Autodesk Inventor part; units mm, degrees
ref_plane "YZ Plane" through (0, 0, 0) normal (1, 0, 0) x (0, 1, 0)
ref_plane "XZ Plane" through (0, 0, 0) normal (0, 1, 0) x (-1, 0, 0)
ref_plane "XY Plane" through (0, 0, 0) normal (0, 0, 1) x (1, 0, 0)
sketch "Sketch1" plane through (0, 0, 0) normal (0, 0, 1) x (1, 0, 0)
  circle A0 centre (0, 0) radius 10
  circle A1 centre (0, 0) radius 20
  line L0 (-15, 0) -> (15, 0)
  line L1 (15, 0) -> (15, 50)
  line L2 (15, 50) -> (-15, 50)
  line L3 (-15, 50) -> (-15, 0)
  point P0 (-15, 13.2288)
  point P1 (15, 13.2288)
  dimension "d0" = 20
  dimension "d1" = 40
  dimension "d2" = 30
  dimension "d3" = 50
extrude "Extrusion1" add sketch "Sketch1" along normal blind 20
sketch "Sketch2" plane through (0, 0, 20) normal (0, 0, 1) x (1, 0, 0)
  circle A0 centre (0, 0) radius 10
  dimension "d6" = 20
extrude "Extrusion2" cut sketch "Sketch2" against normal blind 15
sketch "Sketch4" plane through (-15, 13.2288, 0) normal (-1, 0, 0) x (0, 0, 1)
  line L0 (0, 36.7712) -> (20, 36.7712)
  line L1 (0, 0) -> (0, 36.7712)
  line L2 (20, 36.7712) -> (0, 36.7712)
  line L3 (0, 36.7712) -> (0, 0)
  line L4 (0, 0) -> (20, 0)
  line L5 (20, 0) -> (20, 36.7712)
  line L6 (0, 0) -> (20, 0)
  line L7 (20, 36.7712) -> (10, 36.7712)
  line L8 (10, 36.7712) -> (10, 0)
  line L9 (10, 0) -> (20, 0)
  line L10 (20, 0) -> (20, 36.7712)
  line L11 (10, 0) -> (16, 0)
  line L12 (16, 0) -> (16, 25)
  line L13 (16, 25) -> (10, 25)
  line L14 (10, 25) -> (10, 0)
  line L15 (10, 25) -> (4, 25)
  line L16 (4, 25) -> (4, 0)
  line L17 (4, 0) -> (10, 0)
  line L18 (10, 0) -> (10, 25)
  line L19 (4, 25) -> (16, 25)
  line L20 (16, 25) -> (16, 30.0005)
  line L21 (16, 30.0005) -> (4, 30.0005)
  line L22 (4, 30.0005) -> (4, 25)
  line L23 (4, 30.0005) -> (16, 30.0005)
  line L24 (16, 30.0005) -> (16, 7.0005)
  line L25 (16, 7.0005) -> (4, 7.0005)
  line L26 (4, 7.0005) -> (4, 30.0005)
  line L27 (10, 7.0005) -> (16, 7.0005)
  line L28 (16, 7.0005) -> (16, 0)
  line L29 (16, 0) -> (10, 0)
  line L30 (10, 0) -> (10, 7.0005)
  point P0 (0, -13.2288)
  dimension "d13" = 6
  dimension "d14" = 25
  dimension "d15" = 6
  dimension "d16" = 23
extrude "Extrusion3" cut sketch "Sketch4" against normal blind 23 contours L21 L20 L13 L8 | L8 L15 L22 L21 | L13 L12 L25 L8 | L8 L25 L16 L15
sketch "Sketch6" plane through (-15, 13.2288, 0) normal (-1, 0, 0) x (0, 0, 1)
  line L0 (4, 7.0005) -> (4, 30.0005)
  line L1 (4, 7.0005) -> (16, 7.0005)
  line L2 (16, 7.0005) -> (16, 2.2005)
  line L3 (16, 2.2005) -> (4, 2.2005)
  line L4 (4, 2.2005) -> (4, 7.0005)
  line L5 (4, 30.0005) -> (16, 30.0005)
  line L6 (16, 30.0005) -> (16, 34.8005)
  line L7 (16, 34.8005) -> (4, 34.8005)
  line L8 (4, 34.8005) -> (4, 30.0005)
  point P0 (0, -13.2288)
  dimension "d19" = 12
  dimension "d20" = 4.8
  dimension "d21" = 4.8
extrude "Extrusion4" cut sketch "Sketch6" against normal blind 16
sketch "Sketch7" plane through (1, 13.2288, 0) normal (-1, 0, 0) x (0, 0, 1)
  line L0 (4, 30.0005) -> (16, 30.0005)
  line L1 (4, 30.0005) -> (10, 30.0005)
  line L2 (10, 30.0005) -> (10, 32.5005)
  line L3 (10, 32.5005) -> (4, 32.5005)
  line L4 (4, 32.5005) -> (4, 30.0005)
  circle A0 centre (10, 32.5005) radius 0.75
  line L5 (16, 7.0005) -> (4, 7.0005)
  line L6 (16, 7.0005) -> (16, 2.2005)
  line L7 (4, 7.0005) -> (16, 7.0005)
  line L8 (16, 7.0005) -> (16, 4.5005)
  line L9 (16, 4.5005) -> (4, 4.5005)
  line L10 (4, 4.5005) -> (4, 7.0005)
  line L11 (10, 4.5005) -> (4, 4.5005)
  line L12 (4, 4.5005) -> (4, 7.0005)
  line L13 (4, 7.0005) -> (10, 7.0005)
  line L14 (10, 7.0005) -> (10, 4.5005)
  circle A1 centre (10, 4.5005) radius 0.75
  point P0 (0, -13.2288)
  dimension "d24" = 2.5
  dimension "d25" = 1.5
  dimension "d26" = 2.5
  dimension "d27" = 1.5
extrude "Extrusion5" cut sketch "Sketch7" against normal blind 8 contours A0 L3 L2 | L2 L3 A0 | A1 L9 L14 | L14 L9 A1 | A1 L9
sketch "Sketch8" plane through (15, 13.2288, 0) normal (1, 0, 0) x (0, 0, -1)
  line L0 (0, 36.7712) -> (0, 0)
  line L1 (-20, 36.7712) -> (-20, 0)
  line L2 (0, 36.7712) -> (-20, 36.7712)
  line L3 (-20, 36.7712) -> (-20, 26.7712)
  line L4 (-20, 26.7712) -> (0, 26.7712)
  line L5 (0, 26.7712) -> (0, 36.7712)
  line L6 (0, 26.7712) -> (-20, 26.7712)
  line L7 (-20, 26.7712) -> (-20, 18.7712)
  line L8 (-20, 18.7712) -> (0, 18.7712)
  line L9 (0, 18.7712) -> (0, 26.7712)
  line L10 (0, 26.7712) -> (-10, 26.7712)
  line L11 (-10, 26.7712) -> (-10, 18.7712)
  line L12 (-10, 18.7712) -> (0, 18.7712)
  line L13 (0, 18.7712) -> (0, 26.7712)
  line L14 (-10, 26.7712) -> (-5, 26.7712)
  line L15 (-5, 26.7712) -> (-5, 22.7712)
  line L16 (-5, 22.7712) -> (-10, 22.7712)
  line L17 (-10, 22.7712) -> (-10, 26.7712)
  line L18 (-10, 22.7712) -> (-15, 22.7712)
  line L19 (-15, 22.7712) -> (-15, 26.7712)
  line L20 (-15, 26.7712) -> (-10, 26.7712)
  line L21 (-10, 26.7712) -> (-10, 22.7712)
  point P0 (0, -13.2288)
  dimension "d30" = 10
  dimension "d31" = 8
  dimension "d32" = 5
  dimension "d33" = 5
extrude "Extrusion6" cut sketch "Sketch8" against normal blind 15.8125 contours L15 L16 L11 L4 | L11 L18 L19 L4
sketch "Sketch9" plane through (0, 0, 5) normal (0, 0, 1) x (1, 0, 0)
  circle A0 centre (0, 0) radius 1
  circle A1 centre (7, 0) radius 1.5
  circle A2 centre (0, 0) radius 1.5
  circle A3 centre (-7, 0) radius 1.5
  dimension "d36" = 2
  dimension "d37" = 3
  dimension "d38" = 3
  dimension "d39" = 3
extrude "Extrusion7" cut sketch "Sketch9" against normal blind 8 contours A0 | A1 | A2 | A3
sketch "Sketch10" plane through (-15, 50, 0) normal (0, 1, 0) x (1, 0, 0)
  line L0 (0, 0) -> (0, -20)
  line L1 (0, 0) -> (29.4792, 0)
  line L2 (29.4792, 0) -> (29.4792, -20)
  line L3 (29.4792, -20) -> (0, -20)
  line L4 (0, -20) -> (0, 0)
  point P0 (15, 0)
extrude "Extrusion8" add sketch "Sketch10" along normal blind 10
sketch "Sketch11" plane through (0, 0, 0) normal (0, 0, -1) x (-1, 0, 0)
  line L0 (15, 13.2288) -> (15, 60)
  line L1 (-15, 13.2288) -> (-15, 50)
  line L2 (15, 60) -> (-15, 60)
  line L3 (-15, 60) -> (-15, 45)
  line L4 (-15, 45) -> (15, 45)
  line L5 (15, 45) -> (15, 60)
  line L6 (15, 45) -> (-15, 45)
  line L7 (-15, 45) -> (-15, 35)
  line L8 (-15, 35) -> (15, 35)
  line L9 (15, 35) -> (15, 45)
  point P0 (0, 0)
  dimension "d47" = 15
  dimension "d48" = 10
sketch "Sketch12" plane through (14.4792, 50, 20) normal (1, 0, 0) x (0, 0, -1)
  line L0 (20, 0) -> (20, 10)
  line L1 (0, 0) -> (20, 0)
  line L2 (20, 0) -> (20, 10)
  line L3 (20, 10) -> (0, 10)
  line L4 (0, 10) -> (0, 0)
  point P0 (20, -50)
extrude "Extrusion9" cut sketch "Sketch12" against normal blind 59.6125
sketch "Sketch13" plane through (-15, 50, 0) normal (0, 1, 0) x (1, 0, 0)
  line L0 (30, 0) -> (30, -20)
  line L1 (0, 0) -> (30, 0)
  line L2 (30, 0) -> (30, -20)
  line L3 (30, -20) -> (0, -20)
  line L4 (0, -20) -> (0, 0)
  point P0 (15, 0)
extrude "Extrusion10" add sketch "Sketch13" along normal blind 10
extrude "Extrusion11" add sketch "Sketch11" along normal blind 10
sketch "Sketch15" plane through (0, 0, 20) normal (0, 0, 1) x (1, 0, 0)
  line L0 (-15, 60) -> (15, 60)
  line L1 (-15, 60) -> (0, 60)
  line L2 (0, 60) -> (0, 35)
  line L3 (0, 35) -> (-15, 35)
  line L4 (-15, 35) -> (-15, 60)
  point P0 (0, 0)
  dimension "d56" = 25
extrude "Extrusion12" add sketch "Sketch15" along normal blind 10
sketch "Sketch16" plane through (0, 0, -10) normal (0, 0, -1) x (-1, 0, 0)
  line L0 (-15, 13.2288) -> (-15, 60)
  line L1 (0, 35) -> (15, 35)
  line L2 (-15, 60) -> (0, 60)
  line L3 (0, 60) -> (0, 35)
  line L4 (0, 35) -> (-15, 35)
  line L5 (-15, 35) -> (-15, 60)
  point P0 (0, 0)
extrude "Extrusion13" cut sketch "Sketch16" against normal blind 10
sketch "Sketch18" plane through (0, 0, 20) normal (0, 0, 1) x (1, 0, 0)
  circle A0 centre (0, 0) radius 10
extrude "Extrusion15" add sketch "Sketch18" against normal blind 16
sketch "Sketch19" plane through (0, 0, 0) normal (0, 0, -1) x (-1, 0, 0)
  circle A0 centre (0, 0) radius 1.5
  circle A1 centre (0, 0) radius 10
  dimension "d72" = 20
extrude "Extrusion16" cut sketch "Sketch19" against normal blind 16
sketch "Sketch20" plane through (0, 0, 4) normal (0, 0, -1) x (-1, 0, 0)
  circle A0 centre (0, 0) radius 1.5
  circle A1 centre (0, 0) radius 1.5
extrude "Extrusion17" cut sketch "Sketch20" against normal blind 30.0375
sketch "Sketch21" plane through (0, 0, 16) normal (0, 0, -1) x (-1, 0, 0)
  circle A0 centre (5, 0) radius 1
  circle A1 centre (-5, 0) radius 1
  point P0 (0, 0)
  dimension "d77" = 2
  dimension "d78" = 2
extrude "Extrusion18" cut sketch "Sketch21" against normal blind 138.2375
chamfer "Chamfer2" distance 8 angle 45 1 edges at (10, 0, 0)
sketch "Sketch33" plane through (15, 13.2288, 20) normal (1, 0, 0) x (0, 0, -1)
  line L0 (5, 26.7712) -> (5, 22.7712)
  line L1 (5, 26.7712) -> (15, 26.7712)
  line L2 (15, 26.7712) -> (15, 34.7712)
  line L3 (15, 34.7712) -> (5, 34.7712)
  line L4 (5, 34.7712) -> (5, 26.7712)
  point P0 (20, -13.2288)
  dimension "d110" = 10
  dimension "d111" = 8
extrude "Extrusion27" cut sketch "Sketch33" against normal blind 7
sketch "Sketch41" plane through (-15, 13.2288, 0) normal (-1, 0, 0) x (0, 0, 1)
  line L0 (30, 21.7712) -> (30, 46.7712)
  line L1 (30, 21.7712) -> (20, 21.7712)
  line L2 (20, 21.7712) -> (20, 48.4389)
  line L3 (20, 48.4389) -> (30, 48.4389)
  line L4 (30, 48.4389) -> (30, 21.7712)
  point P0 (0, -13.2288)
extrude "Extrusion31" cut sketch "Sketch41" against normal blind 36.0375
sketch "Sketch42" plane through (0, 0, -10) normal (0, 0, -1) x (-1, 0, 0)
  line L0 (0, 35) -> (15, 35)
  line L1 (0, 60) -> (0, 35)
  line L2 (15, 35) -> (0, 35)
  line L3 (0, 35) -> (0, 60)
  line L4 (0, 60) -> (15, 60)
  line L5 (15, 60) -> (15, 35)
  point P0 (0, 0)
extrude "Extrusion32" add sketch "Sketch42" along normal blind 5
sketch "Sketch43" plane through (-15, 35, 0) normal (0, -1, 0) x (1, 0, 0)
  line L0 (15, -15) -> (15, 0)
  line L1 (0, 0) -> (15, 0)
  line L2 (15, -15) -> (0, -15)
  line L3 (0, -15) -> (0, 0)
  line L4 (0, 0) -> (15, 0)
  line L5 (15, 0) -> (15, -15)
extrude "Extrusion33" add sketch "Sketch43" along normal blind 10
sketch "Sketch44" plane through (-15, 13.2288, 0) normal (-1, 0, 0) x (0, 0, 1)
  line L0 (16, 2.2005) -> (4, 2.2005)
  line L1 (10, 2.2005) -> (10, 34.6918)
  circle A0 centre (10, 24.0854) radius 8
  line L2 (10, 24.0854) -> (-8, 24.0854)
  circle A1 centre (-8, 24.0854) radius 8
  circle A2 centre (-8, 24.0854) radius 2.5
  point P0 (0, -13.2288)
  dimension "d128" = 16
  dimension "d129" = 18
  dimension "d130" = 16
  dimension "d131" = 5
extrude "Extrusion34" add sketch "Sketch44" along normal blind 6 contours A2
sketch "Sketch45" plane through (-15, 60, 0) normal (0, 1, 0) x (1, 0, 0)
  line L0 (0, 0) -> (0, 15)
  line L1 (0, -20) -> (30, -20)
  line L2 (0, 15) -> (15, 15)
  line L3 (15, 15) -> (15, -20)
  line L4 (15, -20) -> (0, -20)
  line L5 (0, -20) -> (0, 15)
  line L6 (30, -20) -> (30, 0)
  line L7 (15, 0) -> (30, 0)
  line L8 (30, 0) -> (30, -20)
  line L9 (30, -20) -> (15, -20)
  line L10 (15, -20) -> (15, 0)
extrude "Extrusion35" cut sketch "Sketch45" against normal blind 7
sketch "Sketch48" plane through (-21, 37.3142, -8) normal (-1, 0, 0) x (0, 0, 1)
  circle A0 centre (0, 0) radius 2.5
  point P0 (8, -37.3142)
extrude "Extrusion36" add sketch "Sketch48" along normal blind 6
sketch "Sketch49" plane through (-15, 13.2288, 0) normal (-1, 0, 0) x (0, 0, 1)
  line L0 (-15, 39.7712) -> (-15, 11.7712)
  line L1 (20, 39.7712) -> (-15, 39.7712)
  line L2 (-15, 11.7712) -> (0, 11.7712)
  line L3 (0, 11.7712) -> (0, 39.7712)
  line L4 (0, 39.7712) -> (-15, 39.7712)
  line L5 (-15, 39.7712) -> (-15, 11.7712)
  circle A0 centre (-8, 24.0854) radius 2.5
  circle A1 centre (-8, 24.0854) radius 2.5
  point P0 (0, -13.2288)
extrude "Extrusion37" add sketch "Sketch49" along normal blind 3.6
sketch "Sketch53" plane through (-27, 37.3142, -8) normal (-1, 0, 0) x (0, 0, 1)
  circle A0 centre (0, 0) radius 2.5
  circle A1 centre (0, 0) radius 2.25
  point P0 (8, -37.3142)
  dimension "d140" = 4.5
extrude "Extrusion38" cut sketch "Sketch53" against normal blind 8.4
sketch "Sketch55" plane through (-18.6, 13.2288, 0) normal (-1, 0, 0) x (0, 0, 1)
  circle A0 centre (-8, 24.0854) radius 2.25 construction
  line L0 (-8, 24.0854) -> (28.6, 24.0854) construction
  circle A1 centre (10.3, 24.0854) radius 2.6362
  point P0 (0, -13.2288)
  dimension "d149" = 18.3
extrude "Extrusion40" add sketch "Sketch55" against normal up to surface (33.6 mm away)
sketch "Sketch56" plane through (-18.6, 37.3142, 10.3) normal (-1, 0, 0) x (0, 0, 1)
  circle A0 centre (0, 0) radius 2.6362
  point P0 (-10.3, -37.3142)
extrude "Extrusion41" add sketch "Sketch56" along normal blind 4
properties part number "NeWConceptV2.0"
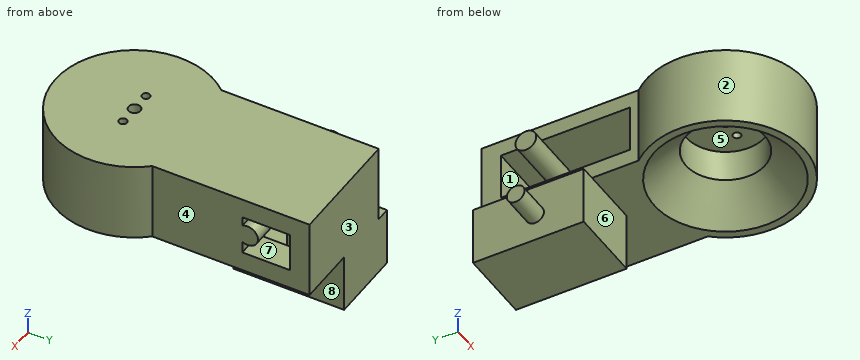
The listing builds one solid part. Answer for the finished solid, in the listing's coordinates (mm). Face numbers are marked on the shaded views. A direction names the side the tool comes from. Give positions to 0.01 mm unless a question says otherwise; leave off trailing zeros. Write each loop counter-clockwise with the first axis right and the second up, starting at its lowest first coordinate (ties: lowest second). Pieces come first, ordered by that corner, then holes.
Item 1: Determine the mould class of the marked faces 6, 7 and 8 for opening direction Y: released by +Y, released by -Y, zero draft, split by the parting line, or undercut.
Item 2: Flat-ended cylindrical pins translate along their axes: P1, Ø4, axis at y = 45.5, z = 10.5, coming from the +X side; P2, Ø5.5, axis at x = 3.5, z = 11, coming from the -Y side; P3, Ø3.5, axis at x = 10.5, z = 11, coming from the -Y side. Find the tip coordinate at first contact, or state that the pin passes through.
Item 3: Section A-A, the plane z = 10 is taken. Write down the section's boundary in (x, y), plus the area to 3 significant figures.
Item 4: Section C-C, the plane z = 1 is taken. Write down the section's boundary in (x, y).
Item 5: Section D-D, the plane x = 5 is taken. Count the separate pieces of the cut face and the enclosed holes in it, plus the area to 3 significant figures.
Item 6: Which of the six approach directions +Z, -Z, +X, -X, +Y, -Y give full straight-line access (tool end or side, diameter ignored) to the marked faces 1, 2, 3, 4 and 5?
Item 7: Find the intervals of material crossed by line 1 along Y through (x, z) = (0, 14.25); line 2 along Y through (x, z) = (0, 11.5); line 3 along Y through (x, z) = (0, 18), in increasing order.
Item 8: Section B-B, the plane y = 0 is taken. Write down the section's boundary in (x, z), plus the area to 3 significant figures.
Completed:
1. face 6: released by -Y
1. face 7: undercut
1. face 8: zero draft
2. P1: stops at x = 8
2. P2: stops at y = -19.99
2. P3: stops at y = -17.98
3. outline: (-22.6, 34.7) - (8, 34.7) - (8, 20.23) - (1, 20.23) - (1, 18.48) - (9, 18.48) - (9, 16.98) - (1, 16.98) - (1, 15.43) - (-15, 15.43) - (-15, 13.23) arc R20 ccw (long way) to (15, 13.23) - (15, 39.93) - (-22.6, 39.93) - close; (-15, 48.03) - (1, 48.03) - (1, 46.48) - (8, 46.48) - (8, 48) - (15, 48) - (15, 53) - (-15, 53) - close; (1, 43.23) - (8, 43.23) - (8, 44.98) - (1, 44.98) - close; hole circle Ø20 at (0, 0)
3. area: 1,390 mm2
4. outline: (-15, 13.23) arc R20 ccw (long way) to (15, 13.23) - (15, 53) - (-15, 53) - close; hole circle Ø34 at (0, 0)
5. separate pieces: 3
5. enclosed holes: 3
5. area: 834 mm2
6. face 1: -X
6. face 2: +Z, -Z
6. face 3: +Z, -Z, +X, -X, +Y
6. face 4: +Z, -Z, +X, +Y
6. face 5: -Z
7. line 1: y = -20 to -10, 10 to 15.43, 48.03 to 53
7. line 2: y = -20 to -10, 10 to 15.43, 34.97 to 39.66, 48.03 to 53
7. line 3: y = -20 to -1.5, 1.5 to 53
8. outline: (-20, 0) - (-18, 0) - (-10, 8) - (-10, 16) - (-6, 16) - (-6, 20) - (-20, 20) - close; (-4, 16) - (-1.5, 16) - (-1.5, 20) - (-4, 20) - close; (1.5, 16) - (4, 16) - (4, 20) - (1.5, 20) - close; (6, 16) - (10, 16) - (10, 8) - (18, 0) - (20, 0) - (20, 20) - (6, 20) - close
8. area: 388 mm2
